```python
from build123d import *

# Parameters (mm, degrees)
F0_R     = 2
F0_R_2   = 1
F1_DEPTH = 6
F7_START = -5.001
F7_DEPTH = 10.002
F8_R     = 3


with BuildPart() as f1:
    # F0 (on Right) → F1 (new body, symmetric)
    with BuildSketch(Plane.YZ):
        with BuildLine():
            Line((2.9962476533, -40.15), (4.9937460889, -0.25))
            ThreePointArc((4.9937460889, -0.25), (0, 5), (-4.9937460889, -0.25))
            Line((-4.9937460889, -0.25), (-2.9962476533, -40.15))
            ThreePointArc((-2.9962476533, -40.15), (0, -43), (2.9962476533, -40.15))
        make_face()
        with Locations((0, -40)):
            Circle(F0_R, mode=Mode.SUBTRACT)
        Circle(F0_R_2, mode=Mode.SUBTRACT)
    extrude(amount=F1_DEPTH, both=True)

    # F2 (on Front) → F3 (revolve, cut)
    with BuildSketch(Plane.XZ):
        Polygon((2.75, 12.5), (-2.75, 12.5), (-2.75, 3), (-4, 3), (-4, 1.25), (-6, 1.25), (-6, 0), (6, 0), (6, 3), (2.75, 3), align=None)
    revolve(axis=Axis((0, 0, 0), (1, 0, 0)), mode=Mode.SUBTRACT)

    # F4 (on Front) → F5 (revolve, cut)
    with BuildSketch(Plane.XZ):
        Polygon((-2.25, -52.5), (0, -52.5), (2.25, -52.5), (2.25, -42), (6, -42), (6, -40), (-6, -40), (-6, -42), (-2.25, -42), align=None)
    revolve(axis=Axis((0, 0, -40), (1, 0, 0)), mode=Mode.SUBTRACT)

    # F6 (on Front) → F7 (intersect)
    with BuildSketch(Plane.XZ.offset(F7_START)):
        Polygon((-4, -43), (0, -43), (4, -43), (4, -37), (6, -12.5), (6, 5), (0, 5), (-6, 5), (-6, -12.5), (-4, -37), align=None)
    extrude(amount=F7_DEPTH, mode=Mode.INTERSECT)

    # F8
    f8_edges = [f1.edges().sort_by_distance(p)[0] for p in [
        (0, -4.420924, -11.69211),
        (0, 4.420924, -11.69211),
        (0, 3.602981, -28.030517),
        (0, -3.602981, -28.030517),
    ]]
    fillet(f8_edges, radius=F8_R)


solid = f1.part
```
Could you check a few things on this model? Use its own coordinates, in mm. A direction names the side the tool comes from. Round coordinates to 2 decimals unless told otherwise and drop trailing zeros. Loops run counter-clockwise (first coordinate to the right, second up) from the corner with the lowest first, then second, coordinate; pieces in that order, holes last. Notation, with made-up numbers: (4, 31) -> (22, 31) arc R10 cw to (22, 35) -> close; hole circle Ø1 at (33.25, 22). An arc over 180 degrees is marked (long way). Put each result on its own line as item: value.
Q1. I want a section at A-A on z = -38.5. Write out the boundary of the cut face in (x, y), and give its area (3 significant figures).
Checks:
outline: (-4, -3.08) -> (-2.25, -3.08) -> (-2.25, -1.32) -> (-4, -1.32) -> close; (-4, 1.32) -> (-2.25, 1.32) -> (-2.25, 3.08) -> (-4, 3.08) -> close; (2.25, -3.08) -> (4, -3.08) -> (4, -1.32) -> (2.25, -1.32) -> close; (2.25, 1.32) -> (4, 1.32) -> (4, 3.08) -> (2.25, 3.08) -> close
area: 12.3 mm2
Q2. For pin 1 Ø5 at (y, z) = (-0.5, -39.5) entering from -X; pin 2 Ø3 at (y, z) = (1, -0.5) entering from +X; pin 3 Ø1 at (x, y) = (1.5, 1) entering from -Z, each with a flat end and sliding along its axis, tell me the tip position at first contact or that it passes through.
Checks:
pin 1: x = -4
pin 2: x = -4
pin 3: z = -27.52
Q3. Which directions (+Z, -Z, +X, -X, +Y, -Y) give clear straight access to the entire face, cutting with the end or side of a thin tool? Please do faces 1 (the flat face through (6, 0, -6)), 2 (the cylindrical face through (0, 0, -12.5)), 3 (the cylindrical face through (-3.137, 1.847, -40.766)), 4 (the flat face through (-4, 1, 1)), 5 (the flat face through (-4, 1, -38)).
Checks:
face 1: +Z, -Z, +X, +Y, -Y
face 2: +Z
face 3: +X, -X
face 4: +X
face 5: -Z, -X, +Y, -Y
Q4. I want a section at D-D on z = -15. Write out the boundary of the cut face in (x, y), and give its area (3 significant figures).
Checks:
outline: (-5.8, -4.26) -> (-2.75, -4.26) -> (-2.75, -4.19) -> (2.75, -4.19) -> (2.75, -4.26) -> (5.8, -4.26) -> (5.8, 4.26) -> (2.75, 4.26) -> (2.75, 4.19) -> (-2.75, 4.19) -> (-2.75, 4.26) -> (-5.8, 4.26) -> close
area: 98.0 mm2
Q5. Thinking about a two-plate mould opening in Y: for faces 6 (the flat face through (2.75, 0, -5)), 7 (the cylindrical face through (-5.01, 1.22, -0.27)), which applies, pulls with the +Y half, pulls with the -Y half, needs draft (parallel to the pull), parting line crosses it, or undercut?
Checks:
face 6: needs draft
face 7: undercut
Q6. I want a section at B-B on x = 1.5. Write out the boundary of the cut face in (y, z) (3 decimals), and give its area (3 significant figures).
Checks:
outline: (-4.225, -15.601) -> (-3.771, -24.669) arc R3 ccw to (-0.625, -27.516) arc R12.5 cw to (0.625, -27.516) arc R3 ccw to (3.771, -24.669) -> (4.225, -15.601) arc R3 ccw to (0.991, -12.461) arc R12.5 cw to (-0.991, -12.461) arc R3 ccw to start
area: 113 mm2
Q7. I want a section at C-C on y = 0. Give the number of separate pieces and of enclosed holes in the cut face, and give its area (3 significant figures).
Checks:
separate pieces: 5
enclosed holes: 0
area: 291 mm2
Q8. Please list where these lines run through material, in increasing order: line 1 (Y direction, x = -3.6, z = -40); line 2 (X direction, y = 4, z = -5); line 3 (Y direction, x = 4.3, z = 0). Write a range as from..to.
Checks:
line 1: -3..-2, 2..3
line 2: -6..-2.75, 2.75..6
line 3: -5..-3, 3..5
